The listing builds one solid part. Answer for the finished solid, in the listing's coordinates (mm). Face numbers are marked on the shaded views. A direction names the side the tool comes from. Give positions to 0.01 mm unless a question says otherwise; leave off trailing zeros. Write each loop counter-clockwise with the first axis right and the second up, starting at its lowest first coordinate (ties: lowest second). Pieces come first, ordered by that corner, then holes. Notation, with made-up numbers: (30.5, -22.75) - (81.5, -22.75) arc R27 cw to (81.5, 10.25) - close; hole circle Ø4 at (-12.5, 72.5). An arc over 180 degrees is marked (long way). One line per item, written item: value. Start each with the question number.
from build123d import *

# Parameters (mm, degrees)
BOSS_EXTRUDE1_DEPTH = 6
SKETCH2_R           = 1.7
SKETCH2_R_2         = 1.25
SKETCH2_R_3         = 2.2
SKETCH2_W           = 25
SKETCH2_H           = 12
SKETCH2_W_2         = 10
SKETCH2_H_2         = 20
SKETCH2_W_3         = 15
SKETCH2_H_3         = 30
SKETCH2_H_4         = 25
CUT_EXTRUDE1_DEPTH  = 142.548578234
SKETCH3_W           = 8
SKETCH3_H           = 46
SKETCH3_W_2         = 46
SKETCH3_H_2         = 8
BOSS_EXTRUDE2_DEPTH = 23
SKETCH4_R           = 1.7
CUT_EXTRUDE2_DEPTH  = 212.416650243
SKETCH5_R           = 1.7
CUT_EXTRUDE3_DEPTH  = 212.416650243
FILLET1_R           = 10
BOSS_EXTRUDE3_START = 5
SKETCH7_R           = 3
SKETCH7_R_2         = 1.25
BOSS_EXTRUDE3_DEPTH = 5


with BuildPart() as part:
    # Sketch1 → Boss-Extrude1 (new body)
    with BuildSketch(Plane(origin=(0, 0, 0), x_dir=(1, 0, 0), z_dir=(0, 1, 0))):
        with BuildLine():
            Line((97.353237465, -22.854915336), (22.854915336, -97.353237465))
            ThreePointArc((22.854915336, -97.353237465), (0, -100), (-22.854915336, -97.353237465))
            Line((-22.854915336, -97.353237465), (-97.353237465, -22.854915336))
            ThreePointArc((-97.353237465, -22.854915336), (-100, 0), (-97.353237465, 22.854915336))
            Line((-97.353237465, 22.854915336), (-22.854915336, 97.353237465))
            ThreePointArc((-22.854915336, 97.353237465), (0, 100), (22.854915336, 97.353237465))
            Line((22.854915336, 97.353237465), (97.353237465, 22.854915336))
            ThreePointArc((97.353237465, 22.854915336), (100, 0), (97.353237465, -22.854915336))
        make_face()
    extrude(amount=BOSS_EXTRUDE1_DEPTH)

    # Sketch2 → Cut-Extrude1 (cut, through all)
    with BuildSketch(Plane(origin=(0, 6, 0), x_dir=(1, 0, 0), z_dir=(0, 1, 0))):
        with Locations(Location((12.5, 25, 0), (0, 0, 270))):
            Circle(SKETCH2_R)
        with Locations(Location((48.5, 25, 0), (0, 0, 270))):
            Circle(SKETCH2_R)
        with Locations(Location((48.5, 49, 0), (0, 0, 270))):
            Circle(SKETCH2_R)
        with Locations(Location((12.5, 49, 0), (0, 0, 270))):
            Circle(SKETCH2_R)
        with Locations(Location((-49, 39, 0), (0, 0, 270))):
            Circle(SKETCH2_R_2)
        with Locations(Location((0, 39, 0), (0, 0, 270))):
            Circle(SKETCH2_R_2)
        with Locations(Location((-49, -19, 0), (0, 0, 270))):
            Circle(SKETCH2_R_2)
        with Locations(Location((0, -19, 0), (0, 0, 270))):
            Circle(SKETCH2_R_2)
        with Locations(Location((-22.5, 85, 0), (0, 0, 270))):
            Circle(SKETCH2_R)
        with Locations(Location((22.5, 85, 0), (0, 0, 270))):
            Circle(SKETCH2_R)
        with Locations(Location((22.5, 65, 0), (0, 0, 270))):
            Circle(SKETCH2_R)
        with Locations(Location((-22.5, 65, 0), (0, 0, 270))):
            Circle(SKETCH2_R)
        with Locations(Location((-40, -70, 0), (0, 0, 270))):
            Circle(SKETCH2_R_3)
        with Locations(Location((40, -70, 0), (0, 0, 270))):
            Circle(SKETCH2_R_3)
        with Locations(Location((40, 70, 0), (0, 0, 270))):
            Circle(SKETCH2_R_3)
        with Locations(Location((-40, 70, 0), (0, 0, 270))):
            Circle(SKETCH2_R_3)
        with Locations(Location((-70, 0, 0), (0, 0, 270))):
            Circle(SKETCH2_R_3)
        with Locations(Location((70, 0, 0), (0, 0, 270))):
            Circle(SKETCH2_R_3)
        with Locations(Location((7, -14, 0), (0, 0, 270))):
            Circle(SKETCH2_R_3)
        with Locations(Location((7, 14, 0), (0, 0, 90))):
            Circle(SKETCH2_R_3)
        with BuildLine():
            Line((15.75, 20.2), (17.25, 20.2))
            ThreePointArc((17.25, 20.2), (18.95, 18.5), (17.25, 16.8))
            Line((17.25, 16.8), (15.75, 16.8))
            ThreePointArc((15.75, 16.8), (14.05, 18.5), (15.75, 20.2))
        make_face()
        with BuildLine():
            Line((60.6, 20.2), (62.4, 20.2))
            ThreePointArc((62.4, 20.2), (64.1, 18.5), (62.4, 16.8))
            Line((62.4, 16.8), (60.6, 16.8))
            ThreePointArc((60.6, 16.8), (58.9, 18.5), (60.6, 20.2))
        make_face()
        with BuildLine():
            Line((15.75, -44.8), (17.25, -44.8))
            ThreePointArc((17.25, -44.8), (18.95, -46.5), (17.25, -48.2))
            Line((17.25, -48.2), (15.75, -48.2))
            ThreePointArc((15.75, -48.2), (14.05, -46.5), (15.75, -44.8))
        make_face()
        with BuildLine():
            Line((60.6, -44.8), (62.4, -44.8))
            ThreePointArc((62.4, -44.8), (64.1, -46.5), (62.4, -48.2))
            Line((62.4, -48.2), (60.6, -48.2))
            ThreePointArc((60.6, -48.2), (58.9, -46.5), (60.6, -44.8))
        make_face()
        with Locations((-34.718614501, -54.191311461)):
            Rectangle(SKETCH2_W, SKETCH2_H)
        with Locations((57.34405649, 37)):
            Rectangle(SKETCH2_W_2, SKETCH2_H_2)
        with Locations((-66.546441163, 22.630683116)):
            Rectangle(SKETCH2_W_3, SKETCH2_H_3)
        with Locations((68.014377365, -23.609307251)):
            Rectangle(SKETCH2_W_2, SKETCH2_H_4)
    extrude(amount=-CUT_EXTRUDE1_DEPTH, mode=Mode.SUBTRACT)

    # Sketch3 → Boss-Extrude2 (add)
    with BuildSketch(Plane(origin=(0, 6, 0), x_dir=(1, 0, 0), z_dir=(0, 1, 0))):
        with Locations((-80, 0)):
            Rectangle(SKETCH3_W, SKETCH3_H)
        with Locations((0, -80)):
            Rectangle(SKETCH3_W_2, SKETCH3_H_2)
        with Locations((80, 0)):
            Rectangle(SKETCH3_W, SKETCH3_H)
    extrude(amount=BOSS_EXTRUDE2_DEPTH)

    # Sketch4 → Cut-Extrude2 (cut, through all)
    with BuildSketch(Plane.ZY.offset(84)):
        with Locations((-20.5, 26)):
            Circle(SKETCH4_R)
        with Locations((20.5, 26)):
            Circle(SKETCH4_R)
        with Locations((20.5, 10)):
            Circle(SKETCH4_R)
        with Locations((-20.5, 10)):
            Circle(SKETCH4_R)
    extrude(amount=-CUT_EXTRUDE2_DEPTH, mode=Mode.SUBTRACT)

    # Sketch5 → Cut-Extrude3 (cut, through all)
    with BuildSketch(Plane.XY.offset(84)):
        with Locations((-20.5, 26)):
            Circle(SKETCH5_R)
        with Locations((20.5, 26)):
            Circle(SKETCH5_R)
        with Locations((20.5, 10)):
            Circle(SKETCH5_R)
        with Locations((-20.5, 10)):
            Circle(SKETCH5_R)
    extrude(amount=-CUT_EXTRUDE3_DEPTH, mode=Mode.SUBTRACT)

    # Fillet1
    fillet1_edges = [part.edges().sort_by_distance(p)[0] for p in [
        (-80, 6, -23),
        (-80, 6, 23),
        (23, 6, 80),
        (-23, 6, 80),
        (80, 6, -23),
        (80, 6, 23),
    ]]
    fillet(fillet1_edges, radius=FILLET1_R)

    # Sketch7 → Boss-Extrude3 (add)
    # profile 1 of 4: a face of its own
    with BuildSketch(Plane(origin=(0, 6, 0), x_dir=(1, 0, 0), z_dir=(0, 1, 0)).offset(BOSS_EXTRUDE3_START)):
        with Locations(Location((-49, 39, 0), (0, 0, 270))):
            Circle(SKETCH7_R)
        with Locations(Location((-49, 39, 0), (0, 0, 270))):
            Circle(SKETCH7_R_2, mode=Mode.SUBTRACT)
    # profile 2 of 4: a face of its own
    with BuildSketch(Plane(origin=(0, 6, 0), x_dir=(1, 0, 0), z_dir=(0, 1, 0)).offset(BOSS_EXTRUDE3_START)):
        with Locations(Location((0, 39, 0), (0, 0, 270))):
            Circle(SKETCH7_R)
        with Locations(Location((0, 39, 0), (0, 0, 270))):
            Circle(SKETCH7_R_2, mode=Mode.SUBTRACT)
    # profile 3 of 4: a face of its own
    with BuildSketch(Plane(origin=(0, 6, 0), x_dir=(1, 0, 0), z_dir=(0, 1, 0)).offset(BOSS_EXTRUDE3_START)):
        with Locations(Location((0, -19, 0), (0, 0, 270))):
            Circle(SKETCH7_R)
        with Locations(Location((0, -19, 0), (0, 0, 270))):
            Circle(SKETCH7_R_2, mode=Mode.SUBTRACT)
    # profile 4 of 4: a face of its own
    with BuildSketch(Plane(origin=(0, 6, 0), x_dir=(1, 0, 0), z_dir=(0, 1, 0)).offset(BOSS_EXTRUDE3_START)):
        with Locations(Location((-49, -19, 0), (0, 0, 270))):
            Circle(SKETCH7_R)
        with Locations(Location((-49, -19, 0), (0, 0, 270))):
            Circle(SKETCH7_R_2, mode=Mode.SUBTRACT)
    extrude(amount=-BOSS_EXTRUDE3_DEPTH)


solid = part.part
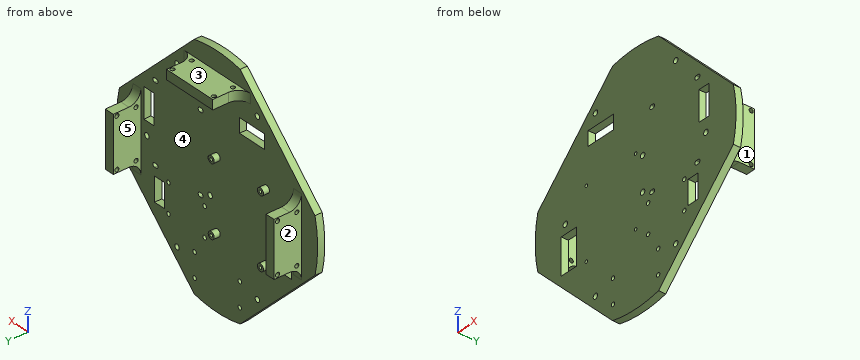
Item 1: Straight lines are drawn through the part: line 1 along X through (y, z) = (3.5, -70); line 2 along X through (y, z) = (12.25, 17); line 3 along X through (y, z) = (1.55, -49). For each, find the intervals that lie inside material, in ascending order.
Item 2: For the marked faces 1, 2, 3, 4 and 5, determine the directions among +Z, -Z, +X, -X, +Y, -Y from which every point of the face is accessible in a straight line to the end or side of a thin tool.
Item 3: Find section B-B on z = 8. Determine the outline of the cut face in (x, y).
Item 4: Find section C-C on z = -78. Determine the outline of the cut face in (x, y).
Item 5: Find section D-D on z = 63. Determine the outline of the cut face in (x, y), plus the area to 3 significant figures.
Item 6: Find section A-A on y = 18.75. Determine the outline of the cut face in (x, z), plus the area to 3 significant figures.
Item 7: Each of these flat-tipped pins is pushed along its axis until it touches: pin 1 Ø10 at (x, z) = (26.5, -44.5) entering from +Y; pin 2 Ø6.5 at (x, y) = (67, 3.5) entering from +Z; pin 3 Ø2.5 at (x, y) = (20.5, 10) entering from +Z; pin 4 Ø5.5 at (x, y) = (20.5, 26) entering from -Z. Where does it stop, or does it pass through?
Values:
1. line 1: -50.21 to -42.2, -37.8 to 37.8, 42.2 to 50.21
1. line 2: -84 to -76, 76 to 84
1. line 3: -71.21 to 10.8, 14.2 to 46.8, 50.2 to 71.21
2. face 1: +Z, -Z, +X, +Y
2. face 2: +Z, -Z, -X, +Y
2. face 3: +Z, +X, -X, +Y
2. face 4: +Y
2. face 5: +Z, -Z, +Y
3. outline: (-99.68, 0) - (99.68, 0) - (99.68, 6) - (84, 6) - (84, 29) - (76, 29) - (76, 6) - (-76, 6) - (-76, 29) - (-84, 29) - (-84, 6) - (-99.68, 6) - close
4. outline: (-42.21, 0) - (42.21, 0) - (42.21, 6) - (-42.21, 6) - close
5. outline: (-57.21, 0) - (57.21, 0) - (57.21, 6) - (-57.21, 6) - close
5. area: 686 mm^2
6. outline: (-84, -23) - (-76, -23) - (-76, 23) - (-84, 23) - close; (-23, 76) - (23, 76) - (23, 84) - (-23, 84) - close; (76, -23) - (84, -23) - (84, 23) - (76, 23) - close
6. area: 1,100 mm^2
7. pin 1: y = 6
7. pin 2: z = 56.46
7. pin 3: through
7. pin 4: z = 76
